```python
from build123d import *

# Parameters (mm, degrees)
BOSS_EXTRUDE2_DEPTH = 6.35
SKETCH3_R           = 3.175
CUT_EXTRUDE1_DEPTH  = 28.679008291
SKETCH1_R           = 3.175
CUT_EXTRUDE2_DEPTH  = 2.54


with BuildPart() as part:
    # Sketch2 → Boss-Extrude2 (new, symmetric)
    with BuildSketch(Plane(origin=(0, 0, 0), x_dir=(1, 0, 0), z_dir=(0, 1, 0))):
        Polygon((-9.525, 0), (9.525, 0), (9.525, -19.05), (3.175, -19.05), (3.175, -6.35), (-3.175, -6.35), (-3.175, -19.05), (-9.525, -19.05), align=None)
    extrude(amount=BOSS_EXTRUDE2_DEPTH, both=True)

    # Sketch3 → Cut-Extrude1 (cut, through all)
    with BuildSketch(Plane.ZY.offset(9.525)):
        with Locations((12.7, 0)):
            Circle(SKETCH3_R)
    extrude(amount=-CUT_EXTRUDE1_DEPTH, mode=Mode.SUBTRACT)

    # Sketch1 → Cut-Extrude2 (cut)
    with BuildSketch(Plane.XY):
        Circle(SKETCH1_R)
    extrude(amount=CUT_EXTRUDE2_DEPTH, mode=Mode.SUBTRACT)


solid = part.part
```
Source: CAD feature listing. Evaluate the final solid. Frame: model axes, mm. A direction names the side the tool comes from. Round coordinates to 2 decimals unless told otherwise and drop trailing zeros. Loops run counter-clockwise (first coordinate to the right, second up) from the corner with the lowest first, then second, coordinate; pieces in that order, holes last. Notation, with made-up numbers: M 40,71 L 94,71 A23 cw 94,89 Z; hole C 74,24 d9. An arc over 180 degrees is marked long. Put each result on its own line as item: value.
(1) First-contact query: pin 1 (5 mm diameter, centred on x = 0, y = 2.5, fed in from +Z); pin 2 (4 mm diameter, centred on x = 0, y = 0, fed in from -Z). Flat tips, straight axial feed; report the tip coordinate or a pass-through.
Solutions:
pin 1: z = 6.35
pin 2: z = 2.54
(2) Ray query, line 1 (X direction, y = -4, z = 17.75) (3 decimals); line 2 (Y direction, x = -6.25, z = 12.7) (3 decimals); line 3 (Z direction, x = -5, y = -2.5). Return the intervals inside material, ascending. Write a range as [from, to].
Solutions:
line 1: [-9.525, -3.175], [3.175, 9.525]
line 2: [-6.35, -3.175], [3.175, 6.35]
line 3: [0, 10.74], [14.66, 19.05]
(3) Section B-B, the plane z = 12.7. Return loops of the section in (x, y) (3 decimals).
Solutions:
outline: M -9.525,-6.35 L -3.175,-6.35 L -3.175,-3.175 L -9.525,-3.175 Z; M -9.525,3.175 L -3.175,3.175 L -3.175,6.35 L -9.525,6.35 Z; M 3.175,-6.35 L 9.525,-6.35 L 9.525,-3.175 L 3.175,-3.175 Z; M 3.175,3.175 L 9.525,3.175 L 9.525,6.35 L 3.175,6.35 Z
(4) Pull-direction query (X, two-part tool) for faces 4 (the face through (-9.525, 2, 10)), 5 (the face through (0, 6.35, 5)), 6 (the face through (-0.69, -3.1, 1.25)); classes: released by +X, released by -X, zero draft, split by the parting line, or undercut.
Solutions:
face 4: released by -X
face 5: zero draft
face 6: undercut
(5) Section D-D, the plane x = 0. Return loops of the section in (y, z) (3 decimals).
Solutions:
outline: M -6.35,0 L -3.175,0 L -3.175,2.54 L 3.175,2.54 L 3.175,0 L 6.35,0 L 6.35,6.35 L -6.35,6.35 Z
(6) Section C-C, the plane y = -4.5. Return loops of the section in (x, z) (3 decimals).
Solutions:
outline: M -9.525,0 L 9.525,0 L 9.525,19.05 L 3.175,19.05 L 3.175,6.35 L -3.175,6.35 L -3.175,19.05 L -9.525,19.05 Z
(7) Section A-A, the plane y = 0. Return loops of the section in (x, z) (3 decimals), and give its area (3 significant figures).
Solutions:
outline: M -9.525,0 L -3.175,0 L -3.175,2.54 L 3.175,2.54 L 3.175,0 L 9.525,0 L 9.525,9.525 L 3.175,9.525 L 3.175,6.35 L -3.175,6.35 L -3.175,9.525 L -9.525,9.525 Z; M -9.525,15.875 L -3.175,15.875 L -3.175,19.05 L -9.525,19.05 Z; M 3.175,15.875 L 9.525,15.875 L 9.525,19.05 L 3.175,19.05 Z
area: 185 mm²
(8) Access query for faces 1 (the face through (6, 0, 19.05)), 2 (the face through (0, 0, 6.35)), 3 (the face through (0, 0, 2.54)). Directions: +Z, -Z, +X, -X, +Y, -Y. A direction counts if a zero-diameter tool reaches every point of the face in a straight line with its end or side. Return the directions, or none.
Solutions:
face 1: +Z, +X, -X, +Y, -Y
face 2: +Z, +Y, -Y
face 3: -Z
